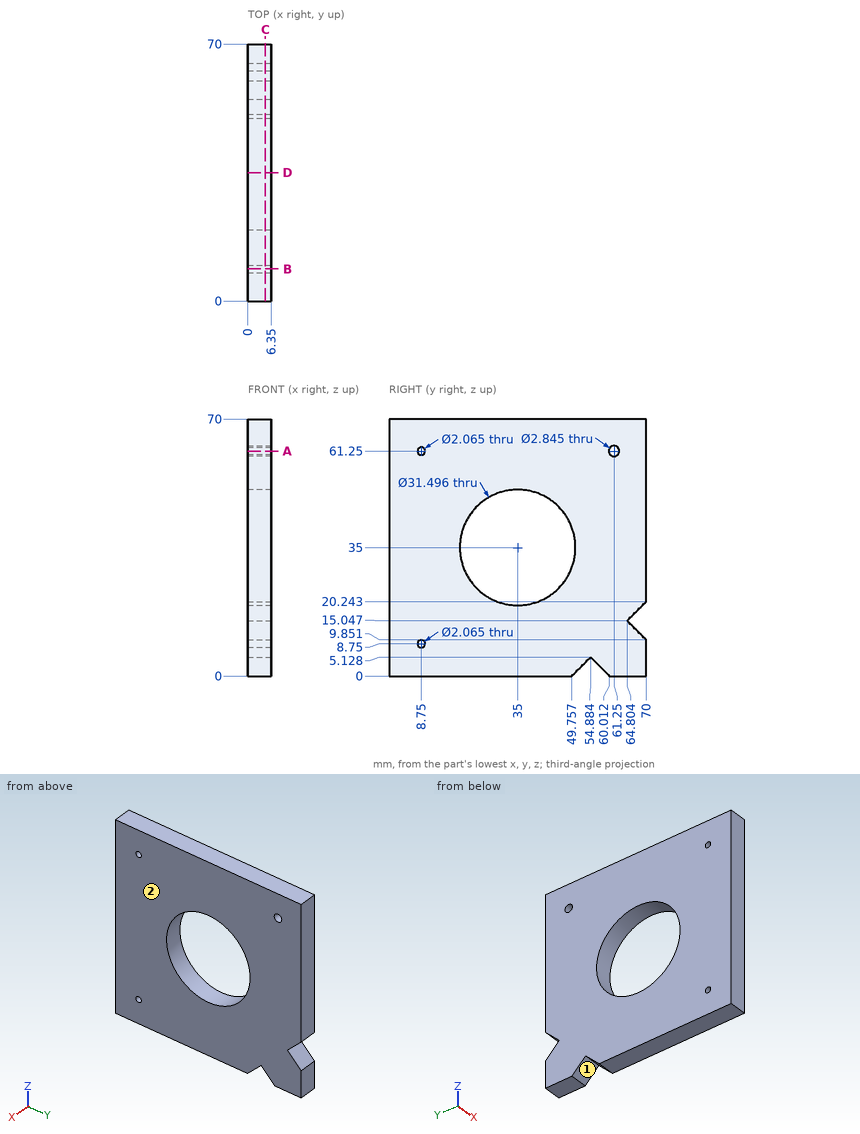
For this review, use the dimensioned drawing (mm, ordinates from the lowest corner) and the shaded views. Coordinates: 2 decimals unless noted, no trailing zeros. Loops run counter-clockwise (first coordinate to the right, second up) from the corner with the lowest first, then second, coordinate; pieces in that order, holes last.
1. For line 1 (Y direction, x = 5, z = 61.25); line 2 (Y direction, x = 1.5, z = 35); line 3 (Y direction, x = 1.5, z = 8.75), list the stretches that pass through material, from the lowest coordinate up.
2. Mouldability with a two-part tool opening along Y and no side actions: class the marked faces 1 and 2 as +Y half, -Y half, draft (parallel to the pull), parting line (faces both ways), or undercut.
3. Add section C-C, the plane x = 4.75. Count the separate pieces of the cut face and the enclosed holes in it, then the cut area to 3 significant figures.
4. Add section B-B, the plane y = 8.75. Give the boundary of the cut face in (x, z).
5. Add section D-D, the plane y = 35. Give the boundary of the cut face in (x, z).
6. Add section A-A, the plane z = 61.25. Give the boundary of the cut face in (x, y).
Result:
1. line 1: y = 0 to 7.72, 9.78 to 59.83, 62.67 to 70
1. line 2: y = 0 to 19.25, 50.75 to 70
1. line 3: y = 0 to 7.72, 9.78 to 70
2. face 1: undercut
2. face 2: draft
3. separate pieces: 1
3. enclosed holes: 4
3. area: 4,050 mm2
4. outline: (0, 0) - (6.35, 0) - (6.35, 7.72) - (0, 7.72) - close; (0, 9.78) - (6.35, 9.78) - (6.35, 60.22) - (0, 60.22) - close; (0, 62.28) - (6.35, 62.28) - (6.35, 70) - (0, 70) - close
5. outline: (0, 0) - (6.35, 0) - (6.35, 19.25) - (0, 19.25) - close; (0, 50.75) - (6.35, 50.75) - (6.35, 70) - (0, 70) - close
6. outline: (0, 0) - (6.35, 0) - (6.35, 7.72) - (0, 7.72) - close; (0, 9.78) - (6.35, 9.78) - (6.35, 59.83) - (0, 59.83) - close; (0, 62.67) - (6.35, 62.67) - (6.35, 70) - (0, 70) - close
